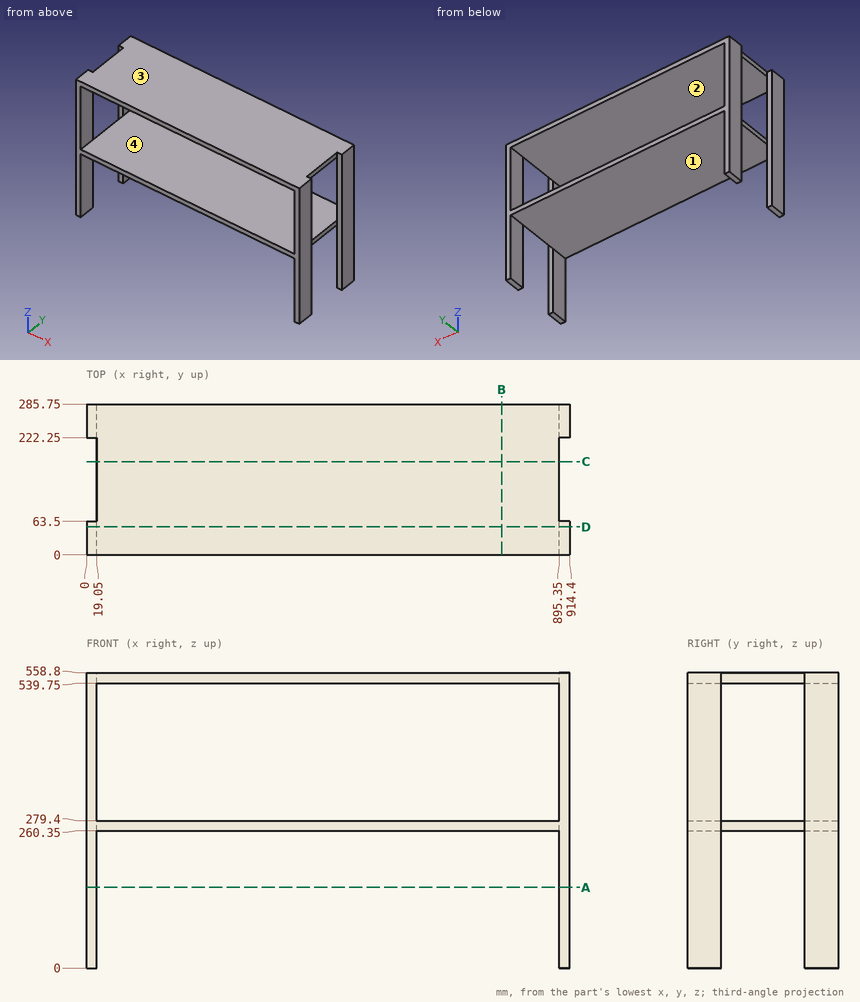
Part print with two shaded views. Sizes in mm from the minimum x, y, z corner. A direction names the side the tool comes from. Coordinates: 2 decimals unless noted, no trailing zeros. Loops run counter-clockwise (first coordinate to the right, second up) from the corner with the lowest first, then second, coordinate; pieces in that order, holes last. Notation, with made-up numbers: M -7.5,21.25 L 18.5,21.25 A27 ccw 18.5,46.25 Z; hole C 32.5,25.25 d1. An arc over 180 degrees is marked long. Use CSV: the item, a comma, the result in double quotes. Start each with the question number.
1. Band-saw the part on A-A, the plane z = 153. List the corners of the cut face in (x, y).
2. Flat gauge pins, fed straight in: pin 1 (15 mm diameter, centred on x = 904, z = 327.5, fed in from -Y); pin 2 (5 mm diameter, centred on x = 155, y = 163, fed in from -Z); pin 3 (15 mm diameter, centred on y = 159, z = 267.5, fed in from +X); pin 4 (21 mm diameter, centred on y = 121.5, z = 549, fed in from -X). Where does each tip first touch, or does it go through?
3. Probe probe 1 along X at (y, z) = (43, 140.5); probe 2 along Z at (x, y) = (820.5, 238). List the from-to ranges inside material, lowest first. Write a range as [from, to].
4. Two-plate mould, pull along X, no slides. Class the marked faces 3 and 4: pulls with the +X half, pulls with the -X half, needs draft (parallel to the pull), parting line crosses it, or undercut.
5. Tool access for the marked faces 1 and 2: list every direction of +Z, -Z, +X, -X, +Y, -Y with a clear straight run to the whole face (end or side of a thin tool).
6. Band-saw the part on C-C, the plane y = 176.5. List the corners of the cut face in (x, z).
7. Band-saw the part on D-D, the plane y = 53. List the corners of the cut face in (x, z), then the cut area to 3 significant figures.
8. Band-saw the part on B-B, the plane x = 786. List the corners of the cut face in (y, z), then the cut area to 3 significant figures.
Entries:
1,outline,"M 0,0 L 19.05,0 L 19.05,63.5 L 0,63.5 Z; M 0,222.25 L 19.05,222.25 L 19.05,285.75 L 0,285.75 Z; M 895.35,0 L 914.4,0 L 914.4,63.5 L 895.35,63.5 Z; M 895.35,222.25 L 914.4,222.25 L 914.4,285.75 L 895.35,285.75 Z"
2,pin 1,"stops at y = 0"
2,pin 2,"stops at z = 260.35"
2,pin 3,"stops at x = 895.35"
2,pin 4,"stops at x = 19.05"
3,probe 1,"x = [0, 19.05], [895.35, 914.4]"
3,probe 2,"z = [260.35, 279.4], [539.75, 558.8]"
4,face 3,"needs draft"
4,face 4,"undercut"
5,face 1,"-Z, +Y, -Y"
5,face 2,"+Y, -Y"
6,outline,"M 19.05,260.35 L 895.35,260.35 L 895.35,279.4 L 19.05,279.4 Z; M 19.05,539.75 L 895.35,539.75 L 895.35,558.8 L 19.05,558.8 Z"
7,outline,"M 0,0 L 19.05,0 L 19.05,260.35 L 895.35,260.35 L 895.35,0 L 914.4,0 L 914.4,558.8 L 0,558.8 Z; hole M 19.05,279.4 L 895.35,279.4 L 895.35,539.75 L 19.05,539.75 Z"
7,area,"54,700 mm2"
8,outline,"M 0,260.35 L 285.75,260.35 L 285.75,279.4 L 0,279.4 Z; M 0,539.75 L 285.75,539.75 L 285.75,558.8 L 0,558.8 Z"
8,area,"10,900 mm2"
